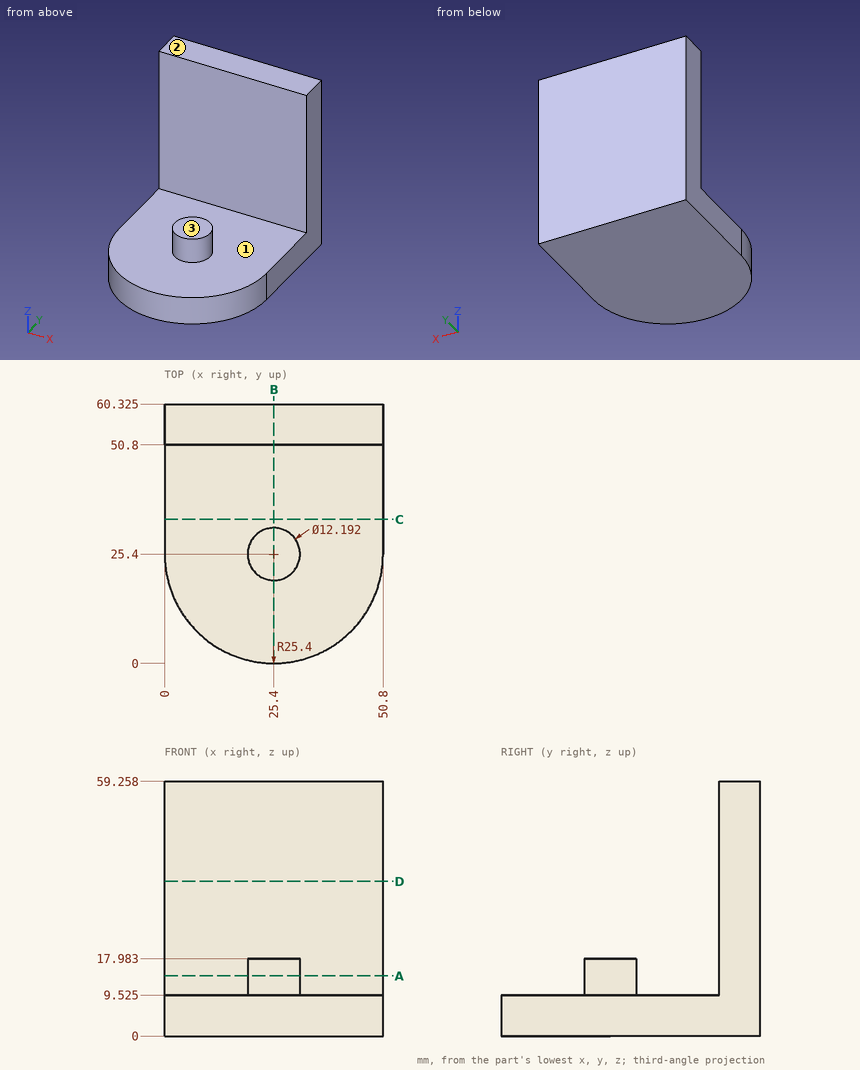
Print and shaded views of the part. All mm, measured from the part's lowest x, y and z. A direction names the side the tool comes from. Round coordinates to 2 decimals unless told otherwise and drop trailing zeros. Loops run counter-clockwise (first coordinate to the right, second up) from the corner with the lowest first, then second, coordinate; pieces in that order, holes last. Notation, with made-up numbers: M -31.75,46 L -2.75,46 A21 ccw -2.75,55 Z; hole C -19,75 d7. An arc over 180 degrees is marked long. One line per question, with ' | ' between items.
1) Flat gauge pins, fed straight in: pin 1 (15 mm diameter, centred on x = 28.5, z = 31.5, fed in from -Y); pin 2 (1 mm diameter, centred on y = 46, z = 10.5, fed in from +X); pin 3 (3.5 mm diameter, centred on x = 24.5, y = 26.5, fed in from +Z). Where does each tip first touch, or does it go through?
Solved:
pin 1: stops at y = 50.8 | pin 2: passes through | pin 3: stops at z = 17.98
2) Band-saw the part on A-A (z = 14). Give the cut face in (x, y) (3 decimals).
Solved:
outline: M 0,50.8 L 50.8,50.8 L 50.8,60.325 L 0,60.325 Z; C 25.4,25.4 d12.192
3) Band-saw the part on C-C (y = 33.5). Give the cut face in (x, z) (3 decimals).
Solved:
outline: M 0,0 L 50.8,0 L 50.8,9.525 L 0,9.525 Z
4) Band-saw the part on D-D (z = 36). Give the cut face in (x, y) (3 decimals), then the cut area to 3 significant figures.
Solved:
outline: M 0,50.8 L 50.8,50.8 L 50.8,60.325 L 0,60.325 Z | area: 484 mm²
5) 3-axis set-ups, long thin cutter, end or side, ignore diameter. For the marked faces 1, 2 and 3: which of +Z, -Z, +X, -X, +Y, -Y reach the whole face in a straight line?
Solved:
face 1: +Z | face 2: +Z, +X, -X, +Y, -Y | face 3: +Z, +X, -X, -Y
6) Drill centre lines: line 1 along Y through (x, z) = (26.5, 27.5) (3 decimals); line 2 along Z through (x, y) = (19.5, 18.5) (3 decimals); line 3 along Z through (x, y) = (22, 27). Where is each one in solid material? Low to high.
Solved:
line 1: y = 50.8 to 60.325 | line 2: z = 0 to 9.525 | line 3: z = 0 to 17.98
7) Band-saw the part on B-B (x = 25.4). Give the cut face in (y, z) (1 decimal), then the cut area to 3 significant figures.
Solved:
outline: M 0,0 L 60.3,0 L 60.3,59.3 L 50.8,59.3 L 50.8,9.5 L 31.5,9.5 L 31.5,18 L 19.3,18 L 19.3,9.5 L 0,9.5 Z | area: 1,150 mm²
